Geometry: final body of the model. Coordinates: model frame, mm. Face numbers are marked on the shaded views. A direction names the side the tool comes from. Round coordinates to 2 decimals unless told otherwise and drop trailing zeros. Order: outer loops, then holes, each group sorted by start corner. A loop starts at its lowest first (then second) coordinate and runs counter-clockwise, first axis right, second up. Notation, with made-up numbers: M -34.5,67.5 L 21.5,67.5 A4 cw 21.5,74.5 Z; hole C -38.75,-5 d7. An arc over 180 degrees is marked long. Put each result on its own line as item: value. Start each with the question number.
1) Material intervals for probe 1 along X at (y, z) = (2, -12.75); probe 2 along Z at (x, y) = (40, 3); probe 3 along Y at (x, z) = (25, -14.5), sorted ascending. Write a range as [from, to].
2) First-contact query: P1, Ø12, axis at x = 11.5, z = -5, coming from the -Y side. Flat tip, straight axial feed; report the tip coordinate or a pass-through.
3) Section A-A, the plane y = 10. Return loops of the section in (x, z), then the cut area to 3 significant figures.
4) Section C-C, the plane y = 30. Return loops of the section in (x, z).
5) Section D-D, the plane x = 25. Return loops of the section in (y, z).
6) Section B-B, the plane z = -4.25. Return loops of the section in (x, y), then the cut area to 3 significant figures.
7) Access query for the marked faces 4 and 5. Directions: +Z, -Z, +X, -X, +Y, -Y. A direction counts if a zero-diameter tool reaches every point of the face in a straight line with its end or side. Return the directions, or none.
8) Draft query along Z for the marked faces 1, 2 and 3. Return one class per face: pulls with the +Z half, pulls with the -Z half, needs draft (parallel to the pull), parting line crosses it, or undercut.
from build123d import *

# Parameters (mm, degrees)
SKETCH1_W                             = 50
SKETCH1_H                             = 20
BOSS_EXTRUDE1_DEPTH                   = 40
M5_CLEARANCE_HOLE1_D                  = 5.5
F_97_0_0059_DIAMETER_HOLE1_AT_2_COUNT = 2
F_97_0_0059_DIAMETER_HOLE1_AT_2_PITCH = 31


with BuildPart() as part:
    # Sketch1 → Boss-Extrude1 (new body)
    with BuildSketch(Plane(origin=(0, 0, 0), x_dir=(1, 0, 0), z_dir=(0, 1, 0))):
        with Locations((25, 10)):
            Rectangle(SKETCH1_W, SKETCH1_H)
    extrude(amount=BOSS_EXTRUDE1_DEPTH)

    # M5 Clearance Hole1 (through all)
    with Locations(Plane.XY):
        with Locations((25, 30), (24.715809074, 10)):
            Hole(M5_CLEARANCE_HOLE1_D / 2)

    # Sketch6 → #97 (0.0059) Diameter Hole1 (revolve, cut)
    with BuildSketch(Plane(origin=(40, 0, -10), x_dir=(0, 0, -1), z_dir=(1, 0, 0))):
        Polygon((0, 0), (0, 14.304540818), (3.8354, 12), (3.8354, 0.71572306), (3.8603936, 0), align=None)
    f_97_0_0059_diameter_hole1 = revolve(axis=Axis((40, -6.35, -10), (0, 1, 0)), mode=Mode.SUBTRACT)

    # #97 (0.0059) Diameter Hole1 at 2: #97 (0.0059) Diameter Hole1 ×2
    with Locations(*[(-i * F_97_0_0059_DIAMETER_HOLE1_AT_2_PITCH, 0, 0) for i in range(1, F_97_0_0059_DIAMETER_HOLE1_AT_2_COUNT)]):
        add(f_97_0_0059_diameter_hole1, mode=Mode.SUBTRACT)


solid = part.part
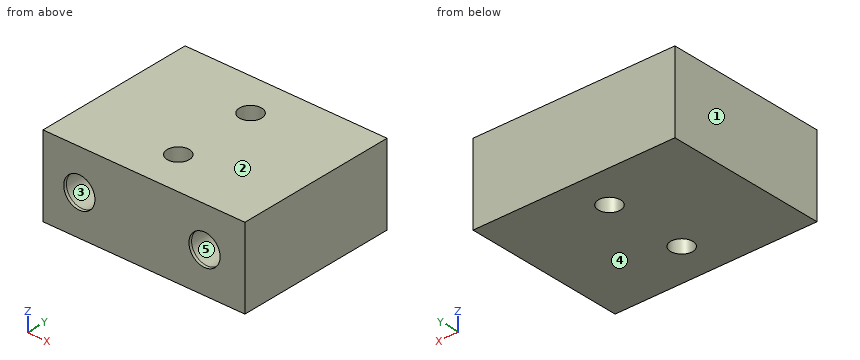
Result sheet:
1. probe 1: x = [0, 6.33], [11.67, 37.33], [42.67, 50]
1. probe 2: z = [-20, -13.84], [-6.16, 0]
1. probe 3: y = [0, 7.26], [12.74, 27.25], [32.75, 40]
2. P1: stops at y = 0
3. outline: M 0,-20 L 21.97,-20 L 21.97,0 L 0,0 Z; M 27.47,-20 L 50,-20 L 50,0 L 27.47,0 Z; hole C 9,-10 d7.67; hole C 40,-10 d7.67
3. area: 798 mm2
4. outline: M 0,-20 L 22.25,-20 L 22.25,0 L 0,0 Z; M 27.75,-20 L 50,-20 L 50,0 L 27.75,0 Z
5. outline: M 0,-20 L 7.26,-20 L 7.26,0 L 0,0 Z; M 12.74,-20 L 27.25,-20 L 27.25,0 L 12.74,0 Z; M 32.75,-20 L 40,-20 L 40,0 L 32.75,0 Z
6. outline: M 0,0 L 50,0 L 50,40 L 0,40 Z; hole C 24.72,10 d5.5; hole C 25,30 d5.5
6. area: 1,950 mm2
7. face 4: -Z, +X, -X, +Y, -Y
7. face 5: -Y
8. face 1: needs draft
8. face 2: pulls with the +Z half
8. face 3: undercut
